```python
from build123d import *

# Parameters (mm, degrees)
SKETCH1_W                      = 211
SKETCH1_H                      = 163
SKETCH1_W_2                    = 176
SKETCH1_H_2                    = 133
BOSS_EXTRUDE1_DEPTH            = 5
CUT_EXTRUDE1_START             = -5
CUT_EXTRUDE1_DEPTH             = 2
CBORE_FOR_M3_SHCS1_D           = 3.4
CBORE_FOR_M3_SHCS1_DEPTH       = 5
CBORE_FOR_M3_SHCS1_CBORE_D     = 6.5
CBORE_FOR_M3_SHCS1_CBORE_DEPTH = 2.68
CHAMFER2_SIZE                  = 1


with BuildPart() as part:
    # Sketch1 → Boss-Extrude1 (new body)
    with BuildSketch(Plane(origin=(0, 0, 0), x_dir=(1, 0, 0), z_dir=(0, 1, 0))):
        with Locations((-2.5, 0)):
            Rectangle(SKETCH1_W, SKETCH1_H)
        Rectangle(SKETCH1_W_2, SKETCH1_H_2, mode=Mode.SUBTRACT)
    extrude(amount=BOSS_EXTRUDE1_DEPTH)

    # Sketch2 → Cut-Extrude1 (cut)
    with BuildSketch(Plane(origin=(0, 5, 0), x_dir=(1, 0, 0), z_dir=(0, 1, 0)).offset(CUT_EXTRUDE1_START)):
        Polygon((-95.75, -71.25), (92.75, -71.25), (92.75, 71.25), (-95.75, 71.25), (-95.75, 10.25), (-102.25, 10.25), (-102.25, 6.75), (-108, 6.75), (-108, -6.75), (-102.25, -6.75), (-102.25, -10.25), (-95.75, -10.25), align=None)
    extrude(amount=CUT_EXTRUDE1_DEPTH, mode=Mode.SUBTRACT)

    # CBORE for M3 SHCS1
    with Locations(Plane(origin=(0, 5, 0), x_dir=(1, 0, 0), z_dir=(0, 1, 0))):
        with Locations((-101.875, 76.375), (0, 76.375), (97.875, 76.375), (97.875, -76.375), (97.875, 0), (0, -76.375), (-101.875, -76.375), (-101.875, -18.25), (-101.875, 18.25)):
            CounterBoreHole(CBORE_FOR_M3_SHCS1_D / 2, CBORE_FOR_M3_SHCS1_CBORE_D / 2, CBORE_FOR_M3_SHCS1_CBORE_DEPTH, depth=CBORE_FOR_M3_SHCS1_DEPTH)

    # Chamfer2
    chamfer2_edges = [part.edges().sort_by_distance(p)[0] for p in [
        (-2.5, 5, 81.5),
        (0, 5, -66.5),
        (-88, 5, 0),
        (0, 5, 66.5),
        (-108, 5, 0),
        (88, 5, 0),
        (-2.5, 5, -81.5),
        (103, 5, 0),
    ]]
    chamfer(chamfer2_edges, length=CHAMFER2_SIZE)


solid = part.part
```
Design review of the part built by this model. Coordinates are the model's own, in mm. A direction names the side the tool comes from. Give positions to 0.01 mm unless a question says otherwise; leave off trailing zeros. Order: outer loops, then holes, each group sorted by start corner. A loop starts at its lowest first (then second) coordinate and runs counter-clockwise, first axis right, second up. Notation, with made-up numbers: (-31.5, 17.25) -> (-18.5, 17.25) arc R12 ccw to (-18.5, 36.25) -> close; hole circle Ø5 at (81, 41.25). An arc over 180 degrees is marked (long way). Write item = value, one per line. Start each with the question number.
(1) To check wall thickness, follow line 1 along X through (y, z) = (1.15, -18); line 2 along X through (y, z) = (1.6, -13); line 3 along Z through (x, y) = (52, 1.3). State the ranges of each line that lie inside material, in increasing order.
(2) For pin 1 (2 mm diameter, centred on x = 99, z = -1, fed in from +Y), flat-tipped, find the tip position at first contact; note if it passes through.
(3) Mouldability with a two-part tool opening along Z and no side actions: class faces 3 (the face through (-8, 2, -69)), 4 (the face through (-11, 0, 72)) as +Z half, -Z half, draft (parallel to the pull), parting line (faces both ways), or undercut.
(4) We need section A-A on x = -55. Write out the cut boundary in (y, z).
(5) For faces 1 (the face through (-3, 5, 71)), 2 (the face through (-100, 2.32, -75)), list the 3-axis set-ups (+Z, -Z, +X, -X, +Y, -Y) from which the entire face can be reached by the end or side of a thin tool; tool diameter is ignored.
(6) We need section B-B on z = 41.5. Write out the cut boundary in (x, y).
(7) We need section C-C on y = 3.1. State how many separate pieces and enclosed holes the cut face has, plus the area to 3 significant figures.
Numbers:
q1.line_1 = -108 to -103.56, -100.19 to -95.75, 92.75 to 103
q1.line_2 = -108 to -95.75, 92.75 to 103
q1.line_3 = -81.5 to -71.25, 71.25 to 81.5
q2.pin_1 = 2.32
q3.face_3 = undercut
q3.face_4 = draft
q4.outline = (0, -81.5) -> (4, -81.5) -> (5, -80.5) -> (5, -67.5) -> (4, -66.5) -> (2, -66.5) -> (2, -71.25) -> (0, -71.25) -> close; (0, 71.25) -> (2, 71.25) -> (2, 66.5) -> (4, 66.5) -> (5, 67.5) -> (5, 80.5) -> (4, 81.5) -> (0, 81.5) -> close
q5.face_1 = +Z, -Z, +X, -X, +Y
q5.face_2 = +Y
q6.outline = (-108, 0) -> (-95.75, 0) -> (-95.75, 2) -> (-88, 2) -> (-88, 4) -> (-89, 5) -> (-107, 5) -> (-108, 4) -> close; (88, 2) -> (92.75, 2) -> (92.75, 0) -> (103, 0) -> (103, 4) -> (102, 5) -> (89, 5) -> (88, 4) -> close
q7.separate_pieces = 1
q7.enclosed_holes = 10
q7.area = 10,700 mm^2
